from build123d import *
from build123d.topology import SkipClean

# Parameters (mm, degrees)
SKETCH3_R            = 27.94
BOSS_EXTRUDE2_DEPTH  = 78
SKETCH5_R            = 3.175
CUT_EXTRUDE1_DEPTH   = 88.437332988
SKETCH4_W            = 14
SKETCH4_H            = 6
SHELL1_START         = 4.5
SHELL1_OUTLINE_R     = 23.44
SHELL1_OUTLINE_R_2   = 7.675
SHELL1_DEPTH         = 6
SHELL1_START_2       = 25.5
SHELL1_2_OUTLINE_R   = 23.44
SHELL1_2_OUTLINE_R_2 = 7.675
SHELL1_2_DEPTH       = 6
SHELL1_START_3       = 46.5
SHELL1_3_OUTLINE_R   = 23.44
SHELL1_3_OUTLINE_R_2 = 7.675
SHELL1_3_DEPTH       = 6
SHELL1_START_4       = 67.5
SHELL1_4_OUTLINE_R   = 23.44
SHELL1_4_OUTLINE_R_2 = 7.675
SHELL1_4_DEPTH       = 6
SHELL1_START_5       = 10.5
SHELL1_5_OUTLINE_R   = 9.44
SHELL1_5_OUTLINE_R_2 = 7.675
SHELL1_5_DEPTH       = 57
BOSS_EXTRUDE3_START  = -73.5
BOSS_EXTRUDE3_DEPTH  = 69
CUT_EXTRUDE3_DEPTH   = 78
BOSS_EXTRUDE5_DEPTH  = 78
SKETCH13_W           = 16.483162312
SKETCH13_H           = 6


# Read off the part's stored shape, not the designer's step: Shell1, Boss-Extrude3
with BuildPart() as part:
    # Sketch3 → Boss-Extrude2 (new body)
    with BuildSketch(Plane.XY):
        Circle(SKETCH3_R)
    extrude(amount=BOSS_EXTRUDE2_DEPTH)

    # Sketch5 → Cut-Extrude1 (cut, through all)
    with BuildSketch(Plane.XY.offset(78)):
        Circle(SKETCH5_R)
    extrude(amount=-CUT_EXTRUDE1_DEPTH, mode=Mode.SUBTRACT)

    # Sketch4 → Cut-Revolve1 (revolve, cut)
    with BuildSketch(Plane(origin=(0, 0, 0), x_dir=(1, 0, 0), z_dir=(0, 1, 0)), mode=Mode.PRIVATE) as cut_revolve1_sk:
        with Locations((-20.94, -60)):
            Rectangle(SKETCH4_W, SKETCH4_H)
        with Locations((-20.94, -39)):
            Rectangle(SKETCH4_W, SKETCH4_H)
        with Locations((-20.94, -18)):
            Rectangle(SKETCH4_W, SKETCH4_H)
    revolve(cut_revolve1_sk.sketch.rotate(Axis((0, 0, 78), (0, 0, -1)), 180), axis=Axis((0, 0, 78), (0, 0, -1)), mode=Mode.SUBTRACT)

    # Shell1 outline → Shell1 (cut)
    with BuildSketch(Plane.XY.offset(SHELL1_START)):
        Circle(SHELL1_OUTLINE_R)
        Circle(SHELL1_OUTLINE_R_2, mode=Mode.SUBTRACT)
    extrude(amount=SHELL1_DEPTH, mode=Mode.SUBTRACT)

    # Shell1 2 outline → Shell1 2 (cut)
    with BuildSketch(Plane.XY.offset(SHELL1_START_2)):
        Circle(SHELL1_2_OUTLINE_R)
        Circle(SHELL1_2_OUTLINE_R_2, mode=Mode.SUBTRACT)
    extrude(amount=SHELL1_2_DEPTH, mode=Mode.SUBTRACT)

    # Shell1 3 outline → Shell1 3 (cut)
    with BuildSketch(Plane.XY.offset(SHELL1_START_3)):
        Circle(SHELL1_3_OUTLINE_R)
        Circle(SHELL1_3_OUTLINE_R_2, mode=Mode.SUBTRACT)
    extrude(amount=SHELL1_3_DEPTH, mode=Mode.SUBTRACT)

    # Shell1 4 outline → Shell1 4 (cut)
    with BuildSketch(Plane.XY.offset(SHELL1_START_4)):
        Circle(SHELL1_4_OUTLINE_R)
        Circle(SHELL1_4_OUTLINE_R_2, mode=Mode.SUBTRACT)
    extrude(amount=SHELL1_4_DEPTH, mode=Mode.SUBTRACT)

    # Shell1 5 outline → Shell1 5 (cut)
    with BuildSketch(Plane.XY.offset(SHELL1_START_5)):
        Circle(SHELL1_5_OUTLINE_R)
        Circle(SHELL1_5_OUTLINE_R_2, mode=Mode.SUBTRACT)
    extrude(amount=SHELL1_5_DEPTH, mode=Mode.SUBTRACT)

    # Boss-Extrude3 outline → Boss-Extrude3 (add)
    with SkipClean():  # the faces are left unmerged after this step: merging them gives an invalid solid
        with BuildSketch(Plane(origin=(0, 0, 0), x_dir=(-1, 0, 0), z_dir=(0, 0, -1)).offset(BOSS_EXTRUDE3_START)):
            with BuildLine():
                ThreePointArc((27.922098775, -1), (27.94, 0), (27.922098775, 1))
                Line((27.922098775, 1), (7.609574561, 1))
                ThreePointArc((7.609574561, 1), (7.675, 0), (7.609574561, -1))
                Line((7.609574561, -1), (27.922098775, -1))
            make_face()
            with BuildLine():
                ThreePointArc((1, 27.922098775), (0, 27.94), (-1, 27.922098775))
                Line((-1, 27.922098775), (-1, 7.609574561))
                ThreePointArc((-1, 7.609574561), (0, 7.675), (1, 7.609574561))
                Line((1, 7.609574561), (1, 27.922098775))
            make_face()
            with BuildLine():
                ThreePointArc((-1, -27.922098775), (0, -27.94), (1, -27.922098775))
                Line((1, -27.922098775), (1, -7.609574561))
                ThreePointArc((1, -7.609574561), (0, -7.675), (-1, -7.609574561))
                Line((-1, -7.609574561), (-1, -27.922098775))
            make_face()
            with BuildLine():
                ThreePointArc((-27.922098775, 1), (-27.94, 0), (-27.922098775, -1))
                Line((-27.922098775, -1), (-7.609574561, -1))
                ThreePointArc((-7.609574561, -1), (-7.675, 0), (-7.609574561, 1))
                Line((-7.609574561, 1), (-27.922098775, 1))
            make_face()
        extrude(amount=BOSS_EXTRUDE3_DEPTH)

    # Sketch16 → Cut-Extrude3 (cut)
    with SkipClean():  # the faces are left unmerged after this step: merging them gives an invalid solid
        with BuildSketch(Plane(origin=(0, 0, 0), x_dir=(-1, 0, 0), z_dir=(0, 0, -1))):
            with BuildLine():
                Line((-3.01340754, -1), (-27.922098775, -1))
                ThreePointArc((-27.922098775, -1), (0, -27.94), (27.922098775, -1))
                Line((27.922098775, -1), (3.01340754, -1))
                ThreePointArc((3.01340754, -1), (0, -3.175), (-3.01340754, -1))
            make_face()
        extrude(amount=-CUT_EXTRUDE3_DEPTH, mode=Mode.SUBTRACT)

    # Sketch18 → Boss-Extrude5 (add)
    with SkipClean():  # the faces are left unmerged after this step: merging them gives an invalid solid
        with BuildSketch(Plane(origin=(0, 0, 0), x_dir=(-1, 0, 0), z_dir=(0, 0, -1))):
            with BuildLine():
                Line((-3.01340754, -1), (-27.922098775, -1))
                Line((-27.922098775, -1), (-27.922098775, -3.5))
                Line((-27.922098775, -3.5), (-6.840431771, -3.5))
                ThreePointArc((-6.840431771, -3.5), (0.000223346, -7.717020739), (6.840632422, -3.49960091))
                Line((6.840632422, -3.49960091), (27.886307794, -3.499359298))
                Line((27.886307794, -3.499359298), (27.922098775, -1))
                Line((27.922098775, -1), (3.01340754, -1))
                ThreePointArc((3.01340754, -1), (0, -3.217020742), (-3.01340754, -1))
            make_face()
        extrude(amount=-BOSS_EXTRUDE5_DEPTH)

    # Sketch13 → Cut-Revolve2 (revolve, cut)
    with BuildSketch(Plane(origin=(0, 0, 0), x_dir=(1, 0, 0), z_dir=(0, 1, 0))):
        with Locations((-22.145666886, -39)):
            Rectangle(SKETCH13_W, SKETCH13_H)
        with Locations((-22.145666886, -18)):
            Rectangle(SKETCH13_W, SKETCH13_H)
        with Locations((-22.145666886, -60)):
            Rectangle(SKETCH13_W, SKETCH13_H)
    revolve(axis=Axis((0, 0, 77.128746248), (0, 0, -1)), mode=Mode.SUBTRACT)


solid = part.part
The listing builds one solid part. Answer for the finished solid, in the listing's coordinates (mm). A direction names the side the tool comes from. Coordinates: 2 decimals unless noted, no trailing zeros. Loops run counter-clockwise (first coordinate to the right, second up) from the corner with the lowest first, then second, coordinate; pieces in that order, holes last.
1) Find section C-C on z = 16.5. Write down the section's boundary in (x, y) (3 decimals).
2) Find section B-B on x = 0. Write down the section's boundary in (y, z) (3 decimals).
3) A tool of negligible diameter and unlimited length cuts with its end or side. For faces 1 (the face through (16.75, 16.4, 49.46)), 2 (the face through (-0.056, -3.217, 38.454)), from which of +Z, -Z, +X, -X, +Y, -Y can it reach the whole face along a straight path? Write none if from no direction.
4) Determine the mould class of faces 3 (the face through (6.74, 6.61, 59.9)), 4 (the face through (0, 10, 78)), 5 (the face through (27.922, -2, 70)), 6 (the face through (-6.61, 6.74, 38.89)) for opening direction Z: pulls with the +Z half, pulls with the -Z half, needs draft (parallel to the pull), parting line crosses it, or undercut.
5) Flat-ended cylindrical pins translate along their axes: pin 1 Ø10 at (x, z) = (-11, 65.5) entering from +Y; pin 2 Ø1.5 at (x, z) = (4.5, 64) entering from -Y; pin 3 Ø1 at (y, z) = (11, 37.5) entering from +X. Find the tip coordinate at first contact, or state that the pin passes through.
6) Find section D-D on x = -16. Give the number of separate pieces and of enclosed holes in the cut face, then the cut area to 3 significant figures.
7) Find the intervals of material crossed by L1, parallel to Z at x = 6.5, y = 25.5; L2, parallel to Z at x = -8, y = 10; L3, parallel to X at y = 0, z = 16 (3 decimals), in increasing order.
Values:
1. outline: (-13.456, -3.5) - (-6.841, -3.5) arc R7.656 ccw to (6.84, -3.5) - (13.456, -3.5) arc R13.904 ccw (long way) to start; hole (-9.387, 1) - (-7.61, 1) arc R7.675 cw to (-1, 7.61) - (-1, 9.387) arc R9.44 ccw to start; hole (-3.013, -1) arc R3.156 ccw to (3.013, -1) arc R3.175 ccw (long way) to start; hole (1, 7.61) arc R7.675 cw to (7.61, 1) - (9.387, 1) arc R9.44 ccw to (1, 9.387) - close
2. outline: (-7.717, 0) - (-3.217, 0) - (-3.217, 78) - (-7.717, 78) - close; (3.175, 0) - (27.94, 0) - (27.94, 15) - (13.904, 15) - (13.904, 21) - (27.94, 21) - (27.94, 36) - (13.904, 36) - (13.904, 42) - (27.94, 42) - (27.94, 57) - (13.904, 57) - (13.904, 63) - (27.94, 63) - (27.94, 78) - (3.175, 78) - close
3. face 1: none
3. face 2: +Z, -Z
4. face 3: undercut
4. face 4: pulls with the +Z half
4. face 5: needs draft
4. face 6: undercut
5. pin 1: stops at y = 27.29
5. pin 2: stops at y = -6.74
5. pin 3: stops at x = 9.11
6. separate pieces: 4
6. enclosed holes: 4
6. area: 1,200 mm2
7. L1: z = 0 to 15, 21 to 36, 42 to 57, 63 to 78
7. L2: z = 0 to 4.5, 10.5 to 25.5, 31.5 to 46.5, 52.5 to 67.5, 73.5 to 78
7. L3: x = -13.904 to -3.175, 3.175 to 13.904
